The listing builds one solid part. Answer for the finished solid, in the listing's coordinates (mm). A direction names the side the tool comes from. Round coordinates to 2 decimals unless told otherwise and drop trailing zeros. Loops run counter-clockwise (first coordinate to the right, second up) from the corner with the lowest first, then second, coordinate; pieces in that order, holes last. Notation, with made-up numbers: (77, 30.25) -> (129, 30.25) arc R22 cw to (129, 48.25) -> close; hole circle Ø7 at (-15, -17.75). An arc over 180 degrees is marked (long way). Use a Markdown table: item, result. Add a question column.
Q1. Section A-A on z = -8.5 is taken. Give the vertices of the cut face in (x, y), then the cut area to 3 significant figures.
Q2. Which of the six approach directions +Z, -Z, +X, -X, +Y, -Y give full straight-line access (tool end or side, diameter ignored) to faces 3 (the cylindrical face through (-19.89, 4.44, 18.52)), 4 (the flat face through (20.87, 6.894, 15.479)), 5 (the flat face through (15, 5, -17)), 6 (the flat face through (22, 8, 0)), 7 (the cylindrical face through (-14.43, 1.48, -11.9))?
Q3. For a pull along X with two mould halves and no side action, classify faces 1 (the flat face through (-24, 13, 0)), 2 (the flat face through (0, 2, -12.5)) as released by +X, released by -X, zero draft, split by the parting line, or undercut.
Q4. Section D-D on x = 18.5 is taken. Give the vertices of the cut face in (y, z), then the cut area to 3 significant figures.
Q5. Given pin 1 Ø3.5 at (x, z) = (18.5, 16) entering from +Y; pin 2 Ø2 at (x, z) = (-8.5, 10.5) entering from +Y (3 decimals), each flat-ended and moving along its own axis, determine where each tip first touches the part or whether it passes through.
Q6. Section C-C on x = 7 is taken. Give the vertices of the cut face in (y, z), then the cut area to 3 significant figures.
Q7. Consider line 1 (X direction, y = 5.5, z = -17.65); line 2 (Y direction, x = -18.5, z = -18.5); line 3 (X direction, y = 12.25, z = 6.5). Determine where each line is inside the solid, lowest interval first.
Q8. Section B-B on y = 12.25 is taken. Give the vertices of the cut face in (x, z).
from build123d import *

# Parameters (mm, degrees)
SKETCH1_W            = 50
SKETCH1_H            = 40
BOSS_EXTRUDE1_DEPTH  = 3
SKETCH2_W            = 30
SKETCH2_H            = 25
CUT_EXTRUDE1_DEPTH   = 4
SKETCH3_W            = 3
SKETCH3_H            = 40
BOSS_EXTRUDE2_DEPTH  = 10
SKETCH4_W            = 7
SKETCH4_H            = 7
BOSS_EXTRUDE3_DEPTH  = 6
SKETCH5_R            = 1.75
CUT_EXTRUDE2_DEPTH   = 41
CUT_EXTRUDE3_DEPTH   = 3
MIRROR3_COPY_1_DEPTH = 3
FILLET1_R            = 3
FILLET2_R            = 2
FILLET3_R            = 2


with BuildPart() as part:
    # Sketch1 → Boss-Extrude1 (new body)
    with BuildSketch(Plane(origin=(0, 0, 0), x_dir=(1, 0, 0), z_dir=(0, 1, 0))):
        Rectangle(SKETCH1_W, SKETCH1_H)
    extrude(amount=BOSS_EXTRUDE1_DEPTH)

    # Sketch2 → Cut-Extrude1 (cut, through all)
    with BuildSketch(Plane(origin=(0, 3, 0), x_dir=(1, 0, 0), z_dir=(0, 1, 0))):
        Rectangle(SKETCH2_W, SKETCH2_H)
    extrude(amount=-CUT_EXTRUDE1_DEPTH, mode=Mode.SUBTRACT)

    # Sketch3 → Boss-Extrude2 (add)
    with BuildSketch(Plane(origin=(0, 3, 0), x_dir=(1, 0, 0), z_dir=(0, 1, 0))):
        with Locations((-23.5, 0)):
            Rectangle(SKETCH3_W, SKETCH3_H)
        with Locations((23.5, 0)):
            Rectangle(SKETCH3_W, SKETCH3_H)
    extrude(amount=BOSS_EXTRUDE2_DEPTH)

    # Sketch4 → Boss-Extrude3 (add)
    with BuildSketch(Plane.XY.offset(20)):
        with Locations((-18.5, 6.5)):
            Rectangle(SKETCH4_W, SKETCH4_H)
        with Locations((18.5, 6.5)):
            Rectangle(SKETCH4_W, SKETCH4_H)
    boss_extrude3 = extrude(amount=-BOSS_EXTRUDE3_DEPTH)

    # Sketch5 → Cut-Extrude2 (cut, through all)
    with BuildSketch(Plane.XY.offset(20)):
        with Locations((-18.5, 5.5)):
            Circle(SKETCH5_R)
        with Locations((18.5, 5.5)):
            Circle(SKETCH5_R)
    cut_extrude2 = extrude(amount=-CUT_EXTRUDE2_DEPTH, mode=Mode.SUBTRACT)

    # Mirror1: Boss-Extrude3, Cut-Extrude2 across plane
    add(boss_extrude3.mirror(Plane.XY))
    add(cut_extrude2.mirror(Plane.XY), mode=Mode.SUBTRACT)

    # Sketch6 → Cut-Extrude3 (cut)
    with BuildSketch(Plane.XY.offset(-14)):
        Polygon((-15.324573519, 5.5), (-16.91228676, 8.25), (-20.08771324, 8.25), (-21.675426481, 5.5), (-20.08771324, 2.75), (-16.91228676, 2.75), align=None)
    cut_extrude3 = extrude(amount=-CUT_EXTRUDE3_DEPTH, mode=Mode.SUBTRACT)

    # Mirror2: Cut-Extrude3 across plane
    add(cut_extrude3.mirror(Plane(origin=(0, 0, 0), x_dir=(0, 0, 1), z_dir=(1, 0, 0))), mode=Mode.SUBTRACT)

    # Mirror3: Cut-Extrude3 across plane
    add(cut_extrude3.mirror(Plane.XY), mode=Mode.SUBTRACT)

    # Mirror3 copy 1 sketch → Mirror3 copy 1 (cut)
    with BuildSketch(Plane(origin=(0, 0, 14), x_dir=(-1, 0, 0), z_dir=(0, 0, -1))):
        Polygon((-15.324573519, 5.5), (-16.91228676, 8.25), (-20.08771324, 8.25), (-21.675426481, 5.5), (-20.08771324, 2.75), (-16.91228676, 2.75), align=None)
    extrude(amount=-MIRROR3_COPY_1_DEPTH, mode=Mode.SUBTRACT)

    # Fillet1
    fillet1_edges = [part.edges().sort_by_distance(p)[0] for p in [
        (-25, 0, 0),
        (25, 0, 0),
    ]]
    fillet(fillet1_edges, radius=FILLET1_R)

    # Fillet2
    fillet2_edges = [part.edges().sort_by_distance(p)[0] for p in [
        (15, 10, -17),
        (-15, 10, 17),
        (15, 10, 17),
        (-15, 10, -17),
    ]]
    fillet(fillet2_edges, radius=FILLET2_R)

    # Fillet3
    fillet3_edges = [part.edges().sort_by_distance(p)[0] for p in [
        (-15, 1.5, 12.5),
        (-15, 1.5, -12.5),
        (15, 1.5, -12.5),
        (15, 1.5, 12.5),
    ]]
    fillet(fillet3_edges, radius=FILLET3_R)


solid = part.part
Checked values:
| question | item | result |
|---|---|---|
| 1 | outline | (-25, 3) arc R3 ccw to (-22, 0) -> (-15, 0) -> (-15, 3) -> (-22, 3) -> (-22, 13) -> (-25, 13) -> close; (15, 0) -> (22, 0) arc R3 ccw to (25, 3) -> (25, 13) -> (22, 13) -> (22, 3) -> (15, 3) -> close |
| 1 | area | 116 mm2 |
| 2 | face 3 | +Z, -Z |
| 2 | face 4 | none |
| 2 | face 5 | +Z, -Z, +Y |
| 2 | face 6 | +Y |
| 2 | face 7 | +Y, -Y |
| 3 | face 1 | zero draft |
| 3 | face 2 | undercut |
| 4 | outline | (0, -20) -> (3.75, -20) -> (3.75, -17) -> (2.75, -17) -> (2.75, -14) -> (3, -14) -> (3, 14) -> (2.75, 14) -> (2.75, 17) -> (3.75, 17) -> (3.75, 20) -> (0, 20) -> close; (7.25, -20) -> (10, -20) -> (10, -14) -> (8.25, -14) -> (8.25, -17) -> (7.25, -17) -> close; (7.25, 17) -> (8.25, 17) -> (8.25, 14) -> (10, 14) -> (10, 20) -> (7.25, 20) -> close |
| 4 | area | 150 mm2 |
| 5 | pin 1 | stops at y = 10 |
| 5 | pin 2 | passes through |
| 6 | outline | (0, -20) -> (3, -20) -> (3, -12.5) -> (0, -12.5) -> close; (0, 12.5) -> (3, 12.5) -> (3, 20) -> (0, 20) -> close |
| 6 | area | 45.0 mm2 |
| 7 | line 1 | x = -25 to -20.25, -16.75 to -15, 15 to 16.75, 20.25 to 25 |
| 7 | line 2 | y = 0 to 3.75, 7.25 to 10 |
| 7 | line 3 | x = -25 to -22, 22 to 25 |
| 8 | outline | (-25, -20) -> (-22, -20) -> (-22, 20) -> (-25, 20) -> close; (22, -20) -> (25, -20) -> (25, 20) -> (22, 20) -> close |
